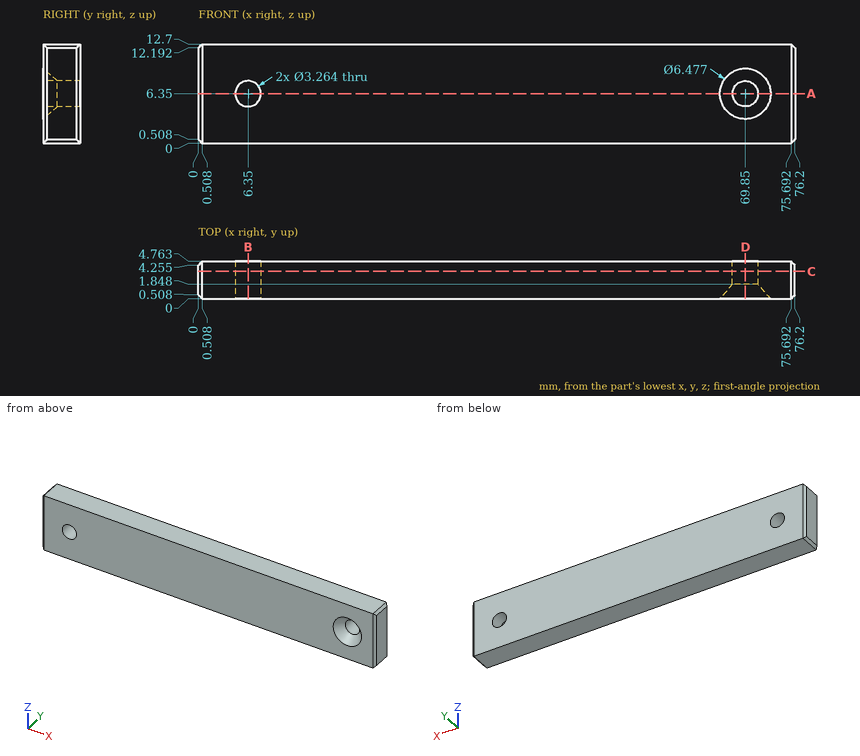
The figure shows three views and two pictorial views of one solid part (mm, origin at its lowest corner). Answer the questions. Give positions to 0.01 mm unless a question says otherwise; leave off trailing zeros. Loops run counter-clockwise (first coordinate to the right, second up) from the corner with the lowest first, then second, coordinate; pieces in that order, holes last. Notation, with made-up numbers: (65.5, -19) -> (75.5, -19) arc R27 ccw to (75.5, 10) -> close; hole circle Ø9 at (2, 48). An arc over 180 degrees is marked (long way). Put each result on its own line as item: value. Start each with the question number.
Item 1: The part is cut by section C-C (y = 3.5). Give the vertices of the cut face in (x, z).
Item 2: The part is cut by section B-B (x = 6.35). Give the vertices of the cut face in (y, z).
Item 3: This flat-tipped pin is pushed along its axis until it touches: P1, Ø4, axis at x = 69.85, z = 6.35, coming from the -Y side (1 decimal). Where does it stop, or does it pass through?
Item 4: The part is cut by section D-D (x = 69.85). Give the vertices of the cut face in (y, z).
Item 5: The part is cut by section A-A (z = 6.35). Give the vertices of the cut face in (x, y) (1 decimal).
Item 6: Find the intervals of material crossed by L1, parallel to Z at x = 69.85, y = 3.1; L2, parallel to X at y = 0.6, z = 7 (1 decimal); L3, parallel to X at y = 3.7, z = 6 (1 decimal), in increasing order. Write a range as [from, to].
Answers below:
1. outline: (0, 0.51) -> (0.51, 0) -> (75.69, 0) -> (76.2, 0.51) -> (76.2, 12.19) -> (75.69, 12.7) -> (0.51, 12.7) -> (0, 12.19) -> close; hole circle Ø3.26 at (6.35, 6.35); hole circle Ø3.26 at (69.85, 6.35)
2. outline: (0, 0) -> (4.76, 0) -> (4.76, 4.72) -> (0, 4.72) -> close; (0, 7.98) -> (4.76, 7.98) -> (4.76, 12.7) -> (0, 12.7) -> close
3. P1: y = 1.4
4. outline: (0, 0) -> (4.76, 0) -> (4.76, 4.72) -> (1.85, 4.72) -> (0, 3.11) -> close; (0, 9.59) -> (1.85, 7.98) -> (4.76, 7.98) -> (4.76, 12.7) -> (0, 12.7) -> close
5. outline: (0, 0.5) -> (0.5, 0) -> (4.7, 0) -> (4.7, 4.8) -> (0.5, 4.8) -> (0, 4.3) -> close; (8, 0) -> (66.6, 0) -> (68.2, 1.8) -> (68.2, 4.8) -> (8, 4.8) -> close; (71.5, 1.8) -> (73.1, 0) -> (75.7, 0) -> (76.2, 0.5) -> (76.2, 4.3) -> (75.7, 4.8) -> (71.5, 4.8) -> close
6. L1: [0, 4.72], [7.98, 12.7]
6. L2: [0, 4.9], [7.8, 67.2], [72.5, 76.2]
6. L3: [0, 4.8], [7.9, 68.3], [71.4, 76.2]
